Part model, mm, in its own coordinate system. Face numbers are marked on the shaded views. A direction names the side the tool comes from. Give positions to 0.01 mm unless a question says otherwise; leave off trailing zeros. Order: outer loops, then holes, each group sorted by start corner. A loop starts at its lowest first (then second) coordinate and runs counter-clockwise, first axis right, second up. Notation, with made-up numbers: M 71.25,69 L 97.25,69 A29 ccw 97.25,92 Z; hole C 84,59.25 d10. An arc over 180 degrees is marked long. Answer as a JSON object with one key per item and string values.
from build123d import *

# Parameters (mm, degrees)
BOSS_EXTRUDE1_DEPTH     = 11.5
SKETCH2_R               = 1.5
CUT_EXTRUDE1_DEPTH      = 1
CUT_EXTRUDE1_DEPTH_BACK = 15.4
FILLET1_R               = 1
FILLET2_R               = 1


with BuildPart() as part:
    # Sketch1 → Boss-Extrude1 (new body, symmetric)
    with BuildSketch(Plane.XY):
        Polygon((-5.2, 1), (5.2, 1), (5.2, 13.5), (7.2, 13.5), (7.2, -1), (-7.2, -1), (-7.2, 13.5), (-5.2, 13.5), align=None)
    extrude(amount=BOSS_EXTRUDE1_DEPTH, both=True)

    # Sketch2 → Cut-Extrude1 (cut, two sides)
    with BuildSketch(Plane(origin=(7.2, 0, 0), x_dir=(0, 0, -1), z_dir=(1, 0, 0))) as cut_extrude1_sk:
        with Locations((-7, 9)):
            Circle(SKETCH2_R)
        with Locations((7, 9)):
            Circle(SKETCH2_R)
    extrude(amount=CUT_EXTRUDE1_DEPTH, mode=Mode.SUBTRACT)
    extrude(cut_extrude1_sk.sketch, amount=-CUT_EXTRUDE1_DEPTH_BACK, mode=Mode.SUBTRACT)

    # Fillet1
    fillet1_edges = [part.edges().sort_by_distance(p)[0] for p in [
        (0, -1, -11.5),
        (0, -1, 11.5),
    ]]
    fillet(fillet1_edges, radius=FILLET1_R)

    # Fillet2
    fillet2_edges = [part.edges().sort_by_distance(p)[0] for p in [
        (-5.2, 1, 0),
        (5.2, 1, 0),
    ]]
    fillet(fillet2_edges, radius=FILLET2_R)


solid = part.part
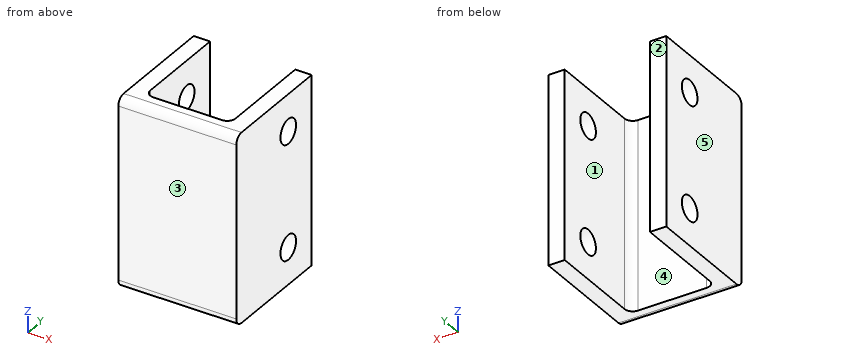
1. Two-plate mould, pull along X, no slides. Class the marked faces 3, 4 and 5: +X half, -X half, draft (parallel to the pull), parting line (faces both ways), or undercut.
Worked answers:
{"face 3": "draft", "face 4": "undercut", "face 5": "-X half"}
2. Probe line 1 along Y through (x, z) = (-5.65, -7); line 2 along X through (y, z) = (11, 8.5); line 3 along Z through (x, y) = (-5.5, 7.75). List the from-to ranges inside material, lowest first.
Worked answers:
{"line 1": "y = -1 to 7.5, 10.5 to 13.5", "line 2": "x = -7.2 to -5.2, 5.2 to 7.2", "line 3": "z = -11.5 to -7.83, -6.17 to 6.17, 7.83 to 11.5"}
3. Which spindle directions (+Z, -Z, +X, -X, +Y, -Y) get a long thin tool onto all of the face, cutting with end or side? Do the marked faces 1 and 2. Say none if no direction does.
Worked answers:
{"face 1": "+Z, -Z, +Y", "face 2": "+Z, -Z, +X, -X, +Y"}
4. Cut at C-C on y = 11. Give the cut face in (x, z).
Worked answers:
{"outline": "M -7.2,-11.5 L -5.2,-11.5 L -5.2,11.5 L -7.2,11.5 Z; M 5.2,-11.5 L 7.2,-11.5 L 7.2,11.5 L 5.2,11.5 Z"}
5. Cut at D-D on x = -2.75. Give the cut face in (y, z).
Worked answers:
{"outline": "M -1,-10.5 A1 ccw 0,-11.5 L 1,-11.5 L 1,11.5 L 0,11.5 A1 ccw -1,10.5 Z"}
6. Cut at B-B on z = -7. Give the cut face in (x, y).
Worked answers:
{"outline": "M -7.2,-1 L 7.2,-1 L 7.2,7.5 L 5.2,7.5 L 5.2,2 A1 cw 4.2,1 L -4.2,1 A1 cw -5.2,2 L -5.2,7.5 L -7.2,7.5 Z; M -7.2,10.5 L -5.2,10.5 L -5.2,13.5 L -7.2,13.5 Z; M 5.2,10.5 L 7.2,10.5 L 7.2,13.5 L 5.2,13.5 Z"}
7. Pin check, flat tip, straight feed: P1, Ø1.5, axis at x = -5, y = 8.5, coming from the -Z side. Stop position of the tip, or through.
Worked answers:
{"P1": "stops at z = -11.5"}
8. Cut at A-A on y = 9. Give the cut face in (x, z).
Worked answers:
{"outline": "M -7.2,-11.5 L -5.2,-11.5 L -5.2,-8.5 L -7.2,-8.5 Z; M -7.2,-5.5 L -5.2,-5.5 L -5.2,5.5 L -7.2,5.5 Z; M -7.2,8.5 L -5.2,8.5 L -5.2,11.5 L -7.2,11.5 Z; M 5.2,-11.5 L 7.2,-11.5 L 7.2,-8.5 L 5.2,-8.5 Z; M 5.2,-5.5 L 7.2,-5.5 L 7.2,5.5 L 5.2,5.5 Z; M 5.2,8.5 L 7.2,8.5 L 7.2,11.5 L 5.2,11.5 Z"}
